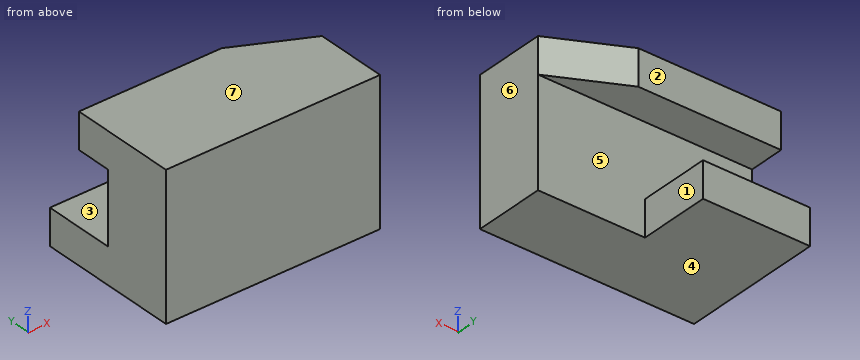
Autodesk Fusion 360 part; units mm, degrees
sketch "Sketch1" plane through (0, 0, 0) normal (0, 1, 0) x (1, 0, 0)
  line L0 (0, 0) -> (60, 0)
  line L1 (60, 0) -> (60, -40)
  line L2 (60, -40) -> (0, -40)
  line L3 (0, -40) -> (0, 0)
  dimension "d1" = 60
  dimension "d2" = 40
extrude "Extrude1" add sketch "Sketch1" along normal blind 20
sketch "Sketch2" plane through (0, 20, 0) normal (0, 1, 0) x (-1, 0, 0)
  line L0 (0, 40) -> (-60, 40)
  line L1 (-60, 40) -> (-60, 0)
  line L2 (-60, 0) -> (0, 0)
  line L3 (0, 0) -> (0, 40)
  line L4 (0, 0) -> (-30, 0)
  line L5 (-30, 0) -> (-30, 10)
  line L6 (-30, 10) -> (0, 10)
  line L7 (0, 10) -> (0, 0)
  dimension "d5" = 30
  dimension "d6" = 10
extrude "Extrude2" add sketch "Sketch2" along normal blind 20 contours L2 L3 L4 L5 L6 L7
sketch "Sketch3" plane through (0, 20, 0) normal (0, 1, 0) x (-1, 0, 0)
  line L0 (-30, 0) -> (-30, 10)
  line L1 (-30, 10) -> (0, 10)
  line L2 (0, 10) -> (0, 40)
  line L3 (0, 40) -> (-60, 40)
  line L4 (-60, 40) -> (-60, 0)
  line L5 (-60, 0) -> (-30, 0)
  line L6 (0, 30) -> (-60, 30)
  line L7 (-60, 30) -> (-60, 40)
  line L8 (-60, 40) -> (0, 40)
  line L9 (0, 40) -> (0, 30)
  dimension "d9" = 10
extrude "Extrude3" add sketch "Sketch3" along normal blind 10 contours L2 L3 L4 L6 L7 L8 L9
sketch "Sketch4" plane through (0, 0, 30) normal (0, 0, -1) x (-1, 0, 0)
  line L0 (-60, 20) -> (0, 20)
  line L1 (0, 20) -> (0, 30)
  line L2 (0, 30) -> (-60, 30)
  line L3 (-60, 30) -> (-60, 20)
  line L4 (-60, 20) -> (-40, 30)
  line L5 (-60, 20) -> (-60, 30)
  line L6 (-40, 30) -> (-60, 30)
  dimension "d12" = 20
extrude "Extrude4" cut sketch "Sketch4" against normal blind 10 contours L2 L3 L4 L5 L6
The model under review builds one solid part; all positions refer to its coordinate system, in mm. Face numbers are marked on the shaded views. A direction names the side the tool comes from. Give positions to 0.01 mm unless a question says otherwise; leave off trailing zeros. Write each loop counter-clockwise with the first axis right and the second up, starting at its lowest first coordinate (ties: lowest second). Pieces come first, ordered by that corner, then holes.
1. Add section A-A, the plane y = 26. Write out the cut boundary in (x, z), plus the area to 3 significant figures.
2. For P1, Ø5, axis at y = 26.5, z = 3, coming from the +X side; P2, Ø11, axis at x = 25, z = 36, coming from the +Y side, all flat-tipped, find the tip position at first contact; note any pin that passes through.
3. Wall thickness on L1, parallel to Z at x = 4, y = 29; L2, parallel to Y at x = 56, z = 28; L3, parallel to Y at x = 25, z = 36.5: over which ranges is each line inside the solid? List them lowest first.
4. Tool access review of the marked faces 1, 2 and 3: name each direction out of +Z, -Z, +X, -X, +Y, -Y from which nothing blocks a thin tool from reaching the whole face with its end or side.
5. Draft analysis for pull direction Z (two halves, no side actions). For the marked faces 4, 5, 6 and 7, state which applies: +Z half, -Z half, draft (parallel to the pull), parting line (faces both ways), or undercut.
6. Add section C-C, the plane y = 21. Write out the cut boundary in (x, z).
7. Add section B-B, the plane x = 10. Write out the cut boundary in (y, z), plus the area to 3 significant figures.
8. Add section D-D, the plane z = 8. Write out the cut boundary in (x, y).
Worked answers:
1. outline: (0, 0) - (30, 0) - (30, 10) - (0, 10) - close; (0, 30) - (48, 30) - (48, 40) - (0, 40) - close
1. area: 780 mm2
2. P1: stops at x = 30
2. P2: stops at y = 30
3. L1: z = 0 to 10, 30 to 40
3. L2: y = 0 to 20
3. L3: y = 0 to 30
4. face 1: -Z, +X, +Y
4. face 2: +Z, +X, -X, +Y
4. face 3: +X, -X, +Y
5. face 4: -Z half
5. face 5: undercut
5. face 6: draft
5. face 7: +Z half
6. outline: (0, 0) - (30, 0) - (30, 10) - (0, 10) - close; (0, 30) - (58, 30) - (58, 40) - (0, 40) - close
7. outline: (0, 0) - (40, 0) - (40, 10) - (20, 10) - (20, 30) - (30, 30) - (30, 40) - (0, 40) - close
7. area: 1,100 mm2
8. outline: (0, 0) - (60, 0) - (60, 20) - (30, 20) - (30, 40) - (0, 40) - close
